Design review of the part shown in the three views and the two pictorial views. Dimensions are in mm from the part's minimum x, y and z. A direction names the side the tool comes from. Give positions to 0.01 mm unless a question says otherwise; leave off trailing zeros. Loops run counter-clockwise (first coordinate to the right, second up) from the corner with the lowest first, then second, coordinate; pieces in that order, holes last. Notation, with made-up numbers: (46.25, 49) -> (99.25, 49) arc R10 ccw to (99.25, 57) -> close; hole circle Ø4 at (44, -35.75). An arc over 180 degrees is marked (long way). Answer as CSV lines item,"result". Start each with the question number.
Item 1: Add section C-C on z = 27.8. State the section outline as (x, y) points.
Item 2: Add section D-D on z = 9. State the section outline as (x, y) points.
Item 3: Clearance check with flat-ended pins moving along their axes: P1, Ø0.9, axis at x = 23, y = 16, coming from the +Z side; P2, Ø8, axis at y = 9.4, z = 27.8, coming from the -X side; P3, Ø8, axis at y = 9.4, z = 76.2, coming from the +X side; P4, Ø3, axis at y = 20.6, z = 76.2, coming from the +X side. State where each tip first meets the part, or that it passes through.
Item 4: For L1, parallel to Y at x = 23.45, z = 27.8; L2, parallel to X at y = 12.75, z = 12; L3, parallel to Z at x = 1.5, y = 18.75, list the stretches that pass through material, from the lowest coordinate up. Write a range as from..to.
Item 5: Add section B-B on y = 20.6. State the section outline as (x, z) points.
Item 6: The part is to be moulded in two halves that separate along X. For the marked faces 1, 2 and 3, say which applies: +X half, -X half, draft (parallel to the pull), parting line (faces both ways), or undercut.
Item 7: Add section A-A on z = 43.5. State the section outline as (x, y) points, plus the area to 3 significant figures.
Item 8: Machinability: for the marked faces 4 and 5, which of the approach directions +Z, -Z, +X, -X, +Y, -Y give a long, thin tool a straight path to every point of the face, cutting with its end or side? Answer none if there is none.
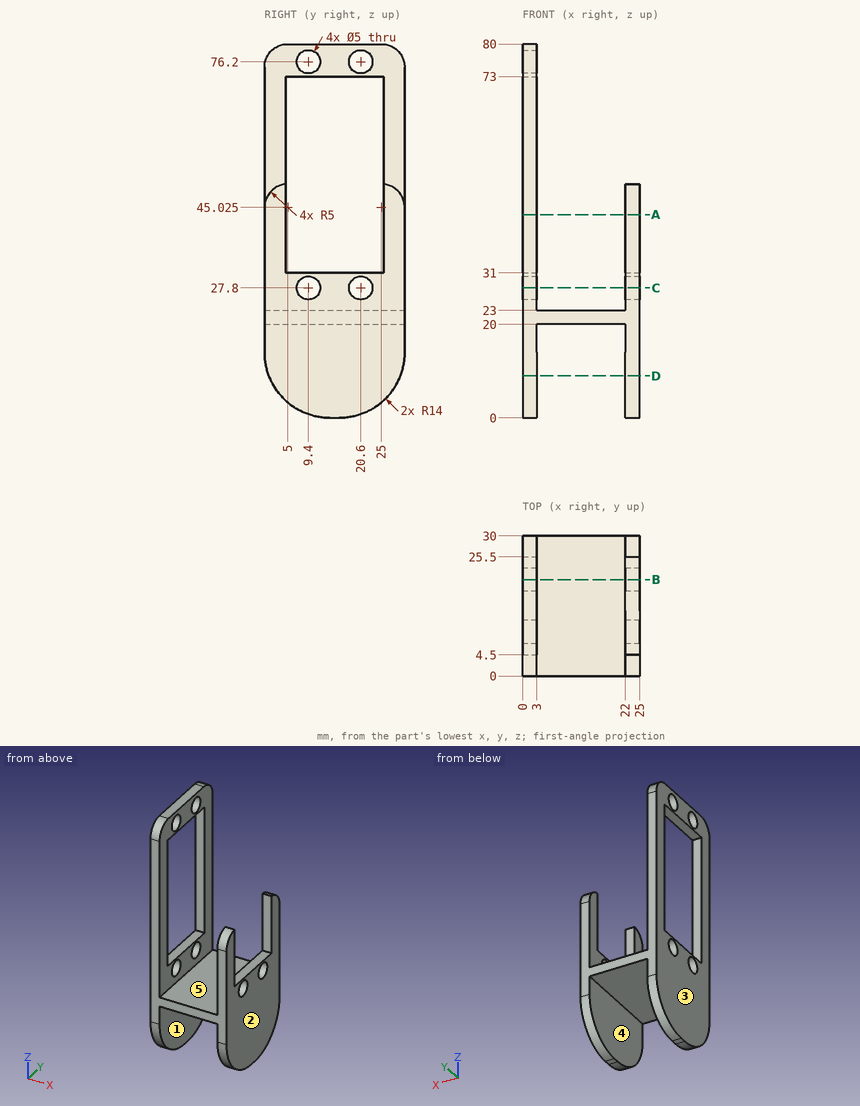
Computed values:
1,outline,"(0, 0) -> (3, 0) -> (3, 6.9) -> (0, 6.9) -> close; (0, 11.9) -> (3, 11.9) -> (3, 18.1) -> (0, 18.1) -> close; (0, 23.1) -> (3, 23.1) -> (3, 30) -> (0, 30) -> close; (22, 0) -> (25, 0) -> (25, 6.9) -> (22, 6.9) -> close; (22, 11.9) -> (25, 11.9) -> (25, 18.1) -> (22, 18.1) -> close; (22, 23.1) -> (25, 23.1) -> (25, 30) -> (22, 30) -> close"
2,outline,"(0, 0.92) -> (3, 0.92) -> (3, 29.08) -> (0, 29.08) -> close; (22, 0.92) -> (25, 0.92) -> (25, 29.08) -> (22, 29.08) -> close"
3,P1,"z = 31"
3,P2,"x = 0"
3,P3,"x = 3"
3,P4,"through"
4,L1,"0..6.9, 11.9..18.1, 23.1..30"
4,L2,"0..3, 22..25"
4,L3,"0.27..26.12, 29.48..31, 73..74.52, 77.88..80"
5,outline,"(0, 0.78) -> (3, 0.78) -> (3, 20) -> (22, 20) -> (22, 0.78) -> (25, 0.78) -> (25, 25.3) -> (22, 25.3) -> (22, 23) -> (3, 23) -> (3, 25.3) -> (0, 25.3) -> close; (0, 30.3) -> (3, 30.3) -> (3, 31) -> (0, 31) -> close; (0, 73) -> (3, 73) -> (3, 73.7) -> (0, 73.7) -> close; (0, 78.7) -> (3, 78.7) -> (3, 80) -> (0, 80) -> close; (22, 30.3) -> (25, 30.3) -> (25, 31) -> (22, 31) -> close"
6,face 1,"undercut"
6,face 2,"+X half"
6,face 3,"-X half"
7,outline,"(0, 0) -> (3, 0) -> (3, 4.5) -> (0, 4.5) -> close; (0, 25.5) -> (3, 25.5) -> (3, 30) -> (0, 30) -> close; (22, 0) -> (25, 0) -> (25, 4.5) -> (22, 4.5) -> close; (22, 25.5) -> (25, 25.5) -> (25, 30) -> (22, 30) -> close"
7,area,"54.0 mm²"
8,face 4,"-Z, +Y, -Y"
8,face 5,"+Z, +Y, -Y"
